```python
from build123d import *

# Parameters (mm, degrees)
F0_R     = 8
F1_DEPTH = 2.5
F2_R     = 2.49999
F3_R     = 1.55
F4_DEPTH = 25
F5_R     = 2.2
F5_R_2   = 1.55
F6_DEPTH = 1.35


# Not quite as in the source:
# - a fillet or chamfer is up to 0.001 mm smaller than in the source, because OpenCascade refuses the exact size


with BuildPart() as f1:
    # F0 (on Front) → F1 (new body)
    with BuildSketch(Plane.XZ):
        Circle(F0_R)
    extrude(amount=F1_DEPTH)

    # F2 (radius 2.5 in the source; OpenCascade refuses exactly that, so slightly less here)
    f2_edges = [f1.edges().sort_by_distance(p)[0] for p in [
        (-8, -2.5, 0),
    ]]
    fillet(f2_edges, radius=F2_R)

    # F3 (on face) → F4 (cut)
    with BuildSketch(Plane(origin=(0, 0, 0), x_dir=(-1, 0, 0), z_dir=(0, 1, 0))):
        Circle(F3_R)
    extrude(amount=-F4_DEPTH, mode=Mode.SUBTRACT)

    # F5 (on face) → F6 (cut)
    with BuildSketch(Plane.XZ.offset(2.5)):
        Circle(F5_R)
        Circle(F5_R_2, mode=Mode.SUBTRACT)
    extrude(amount=-F6_DEPTH, mode=Mode.SUBTRACT)


solid = f1.part
```
Geometry check sheet. Reference: the model listing, model coordinates, mm. A direction names the side the tool comes from. Give positions to 0.01 mm unless a question says otherwise; leave off trailing zeros. Order: outer loops, then holes, each group sorted by start corner. A loop starts at its lowest first (then second) coordinate and runs counter-clockwise, first axis right, second up.
1. Gauge pin test, flat ends, axial feed: pin 1 Ø6 at (x, z) = (-4, 5.5) entering from +Y; pin 2 Ø4 at (x, z) = (0, 0) entering from -Y. Record the tip position at first contact, or that the pin passes through.
2. Release check for a two-part mould opening along Z. For faces 1 (the face through (-0.715, -0.567, -1.375)), 2 (the face through (2, 0, 0)) record: pulls with the +Z half, pulls with the -Z half, needs draft (parallel to the pull), parting line crosses it, or undercut.
3. Thickness scan on L1, parallel to X at y = -0.9, z = -0.25; L2, parallel to Z at x = 0, y = -0.9; L3, parallel to X at y = -2.1, z = -0.5. Record the ranges inside material, lowest first.
4. Section check D-D, the plane y = -2.3. Enter the section's corners in (x, z).
5. Access from +Z, -Z, +X, -X, +Y, -Y to the whole of each face (thin tool, end or side, straight path). Record for faces 3 (the face through (0.95, -1.15, -1.44)), 4 (the face through (2.4, -2.5, 0.1)).
6. Section check C-C, the plane y = -0.35. Enter the section's corners in (x, z), and give its area (3 significant figures).
Values follow:
1. pin 1: stops at y = 0
1. pin 2: stops at y = -1.15
2. face 1: undercut
2. face 2: needs draft
3. L1: x = -7.83 to -1.53, 1.53 to 7.83
3. L2: z = -7.83 to -1.55, 1.55 to 7.83
3. L3: x = -6.84 to -2.14, 2.14 to 6.84
4. outline: circle Ø12.96 at (0, 0); hole circle Ø4.4 at (0, 0)
5. face 3: -Y
5. face 4: +Z, -Z, +X, -X, -Y
6. outline: circle Ø15.95 at (0, 0); hole circle Ø3.1 at (0, 0)
6. area: 192 mm2
